Geometry: final body of the model. Coordinates: model frame, mm. A direction names the side the tool comes from. Give positions to 0.01 mm unless a question says otherwise; leave off trailing zeros. Loops run counter-clockwise (first coordinate to the right, second up) from the corner with the lowest first, then second, coordinate; pieces in that order, holes last. Notation, with made-up numbers: (67, 36.5) -> (116, 36.5) arc R19 cw to (116, 69.5) -> close; hole circle Ø11 at (14, 27). An arc over 180 degrees is marked (long way). Answer in a Markdown table with one row per item. Add a question column.
1) Draft query along X for faces 1 (the cylindrical face through (14.29, -7.97, 2.54)), 2 (the flat face through (0, 0, 0)), 3 (the flat face through (22.5, 0, 2)), 4 (the cylindrical face through (-19.5, -9.9, 2.5)). Return one class per face: +X half, -X half, draft (parallel to the pull), parting line (faces both ways), or undercut.
2) Section query C-C (x = -16.5). Return the cut outline in (y, z), plus the area to 3 significant figures.
3) First-contact query: P1, Ø11.5, axis at y = -6.5, z = 16.5, coming from the +X side; P2, Ø2, axis at x = -8.5, y = -0.5, coming from the +Z side; P3, Ø6, axis at y = -8, z = 22, coming from the -X side. Flat tips, straight axial feed; report the tip coordinate or a pass-through.
4) Line query: line 1 (Y direction, x = 16.5, z = 1.05); line 2 (Y direction, x = -2.5, z = 19); line 3 (X direction, y = -12, z = 4.75). Output: solid intervals per line, ascending. Write a range as from..to.
5) Access query for faces 5 (the flat face through (13, 0, 5)), 6 (the flat face through (-13, 0, 5)), 7 (the cylindrical face through (-19.5, 0.1, 2.5)). Directions: +Z, -Z, +X, -X, +Y, -Y. A direction counts if a zero-diameter tool reaches every point of the face in a straight line with its end or side. Return the directions, or none.
6) Section query B-B (y = 0). Return the cut outline in (x, z).
7) Section query D-D (z = 19). Return the cut outline in (x, y), plus the area to 3 significant figures.
8) Section query A-A (z = 4.5). Return the cut outline in (x, y).
```python
from build123d import *

# Parameters (mm, degrees)
SKETCH1_W           = 45
SKETCH1_H           = 30
BASE_DEPTH          = 5
SKETCH2_W           = 10
SKETCH2_H           = 30
BOSS_EXTRUDE2_DEPTH = 25
SKETCH3_R           = 7
CUT_EXTRUDE3_DEPTH  = 10
SKETCH9_R           = 3
SCREW_DEPTH         = 5
FILLET1_R           = 2
FILLET2_R           = 2


with BuildPart() as part:
    # Sketch1 → Base (new body)
    with BuildSketch(Plane.XY):
        Rectangle(SKETCH1_W, SKETCH1_H)
    extrude(amount=BASE_DEPTH)

    # Sketch2 → Boss-Extrude2 (add)
    with BuildSketch(Plane.XY.offset(5)):
        Rectangle(SKETCH2_W, SKETCH2_H)
    extrude(amount=BOSS_EXTRUDE2_DEPTH)

    # Sketch3 → Cut-Extrude3 (cut)
    with BuildSketch(Plane.ZY.offset(5)):
        with Locations((19, 0)):
            Circle(SKETCH3_R)
    extrude(amount=-CUT_EXTRUDE3_DEPTH, mode=Mode.SUBTRACT)

    # Sketch9 → Screw (cut)
    with BuildSketch(Plane.XY.offset(5)):
        with Locations((-16.5, 10)):
            Circle(SKETCH9_R)
        with Locations((-16.5, 0)):
            Circle(SKETCH9_R)
        with Locations((-16.5, -10)):
            Circle(SKETCH9_R)
        with Locations((16.5, -10)):
            Circle(SKETCH9_R)
        with Locations((16.5, 0)):
            Circle(SKETCH9_R)
        with Locations((16.5, 10)):
            Circle(SKETCH9_R)
    extrude(amount=-SCREW_DEPTH, mode=Mode.SUBTRACT)

    # Fillet1
    fillet1_edges = [part.edges().sort_by_distance(p)[0] for p in [
        (-5, 0, 5),
    ]]
    fillet(fillet1_edges, radius=FILLET1_R)

    # Fillet2
    fillet2_edges = [part.edges().sort_by_distance(p)[0] for p in [
        (5, 0, 5),
    ]]
    fillet(fillet2_edges, radius=FILLET2_R)


solid = part.part
```
Evaluation:
| question | item | result |
|---|---|---|
| 1 | face 1 | undercut |
| 1 | face 2 | draft |
| 1 | face 3 | +X half |
| 1 | face 4 | undercut |
| 2 | outline | (-15, 0) -> (-13, 0) -> (-13, 5) -> (-15, 5) -> close; (-7, 0) -> (-3, 0) -> (-3, 5) -> (-7, 5) -> close; (3, 0) -> (7, 0) -> (7, 5) -> (3, 5) -> close; (13, 0) -> (15, 0) -> (15, 5) -> (13, 5) -> close |
| 2 | area | 60.0 mm² |
| 3 | P1 | x = 5 |
| 3 | P2 | z = 5 |
| 3 | P3 | x = -5 |
| 4 | line 1 | -15..-13, -7..-3, 3..7, 13..15 |
| 4 | line 2 | -15..-7, 7..15 |
| 4 | line 3 | -22.5..-18.74, -14.26..14.26, 18.74..22.5 |
| 5 | face 5 | +Z, +X, +Y, -Y |
| 5 | face 6 | +Z, -X, +Y, -Y |
| 5 | face 7 | +Z, -Z |
| 6 | outline | (-22.5, 0) -> (-19.5, 0) -> (-19.5, 5) -> (-22.5, 5) -> close; (-13.5, 0) -> (13.5, 0) -> (13.5, 5) -> (7, 5) arc R2 cw to (5, 7) -> (5, 12) -> (-5, 12) -> (-5, 7) arc R2 cw to (-7, 5) -> (-13.5, 5) -> close; (-5, 26) -> (5, 26) -> (5, 30) -> (-5, 30) -> close; (19.5, 0) -> (22.5, 0) -> (22.5, 5) -> (19.5, 5) -> close |
| 7 | outline | (-5, -15) -> (5, -15) -> (5, -7) -> (-5, -7) -> close; (-5, 7) -> (5, 7) -> (5, 15) -> (-5, 15) -> close |
| 7 | area | 160 mm² |
| 8 | outline | (-22.5, -15) -> (22.5, -15) -> (22.5, 15) -> (-22.5, 15) -> close; hole circle Ø6 at (-16.5, -10); hole circle Ø6 at (-16.5, 0); hole circle Ø6 at (-16.5, 10); hole circle Ø6 at (16.5, -10); hole circle Ø6 at (16.5, 0); hole circle Ø6 at (16.5, 10) |
